Here's how the part is built. I have some questions about the finished solid (model axes, mm). A direction names the side the tool comes from. Coordinates: 2 decimals unless noted, no trailing zeros. Write each loop counter-clockwise with the first axis right and the second up, starting at its lowest first coordinate (ties: lowest second). Pieces come first, ordered by that corner, then holes.
(1) Imagine slicing it at B-B, the plane y = 72. List the corners of the cut face in (x, z) for me, plus the area to 3 significant figures.
(2) Imagine slicing it at A-A, the plane z = -4. List the corners of the cut face in (x, y) for me.
(3) Thinking about a two-plate mould opening in Y: for faces 1 (the cylindrical face through (-15.07, -64.7, 2.99)), 2 (the flat face through (-20, -18, -4)), 3 (the flat face through (15, -40, -6)), which applies, released by +Y, released by -Y, zero draft, split by the parting line, or undercut?
(4) For pin 1 Ø3 at (x, y) = (-17, -43) entering from -Z; pin 2 Ø20 at (x, y) = (-9.5, 35) entering from -Z; pin 3 Ø3 at (x, z) = (-5.5, -50.5) entering from -Y, each with a flat end and sliding along its axis, tell me the tip position at first contact or that it passes through.
(5) Imagine slicing it at C-C, the plane x = 0. List the corners of the cut face in (y, z) for me, plus the area to 3 significant figures.
(6) Imagine slicing it at D-D, the plane z = -20. List the corners of the cut face in (x, y) for me.
(7) Which directions (+Z, -Z, +X, -X, +Y, -Y) give clear straight access to the entire face, cutting with the end or side of a thin tool? Please do faces 4 (the flat face through (2, 55, 9)), 5 (the flat face through (20, -19, -4)), 6 (the flat face through (-10, -35.5, -6.4)), 7 (the flat face through (15, -41, 6)), 8 (the cylindrical face through (0, 20, 10)).
(8) Please list where these lines run through material, in increasing order: probe 1 along X at (y, z) = (0, -31); probe 2 along X at (y, z) = (-8, 4).
```python
from build123d import *

# Parameters (mm, degrees)
BOSS_EXTRUDE1_DEPTH      = 9
BOSS_EXTRUDE2_DEPTH      = 6
BOSS_EXTRUDE3_DEPTH      = 15
BOSS_EXTRUDE3_DEPTH_BACK = 70
SKETCH1_4_R              = 20
BOSS_EXTRUDE4_DEPTH      = 10
SKETCH3_W                = 10
SKETCH3_H                = 85.001


with BuildPart() as part:
    # Sketch1 → Boss-Extrude1 (new, symmetric)
    with BuildSketch(Plane.XY):
        with BuildLine():
            ThreePointArc((-29.862613088, 88), (2.137386912, 56), (34.137386912, 88))
            Line((34.137386912, 88), (42.137386912, 88))
            ThreePointArc((42.137386912, 88), (2.137386912, 48), (-37.862613088, 88))
            Line((-37.862613088, 88), (-29.862613088, 88))
        make_face()
    extrude(amount=BOSS_EXTRUDE1_DEPTH, both=True)

    # Sketch1<3> → Boss-Extrude2 (add, symmetric)
    with BuildSketch(Plane.XY):
        with BuildLine():
            ThreePointArc((20, 52.209958736), (-0.332230393, 48.076310411), (-20, 54.684296485))
            Line((-20, 54.684296485), (-20, 0))
            ThreePointArc((-20, 0), (0, 20), (20, 0))
            Line((20, 0), (20, 52.209958736))
        make_face()
    extrude(amount=BOSS_EXTRUDE2_DEPTH, both=True)

    # Sketch1<4> → Boss-Extrude3 (add, two sides: drawn at the far end of the back side and taken through both)
    with BuildSketch(Plane.XY.offset(-BOSS_EXTRUDE3_DEPTH_BACK)):
        Circle(SKETCH1_4_R)
    extrude(amount=BOSS_EXTRUDE3_DEPTH + BOSS_EXTRUDE3_DEPTH_BACK)

    # Sketch2 → Boss-Extrude4 (add)
    with BuildSketch(Plane(origin=(20, 0, 0), x_dir=(0, 0, -1), z_dir=(1, 0, 0))):
        with BuildLine():
            Line((-15, 0), (-15, -50))
            ThreePointArc((-15, -50), (-2.703242507, -64.754405442), (14.025663993, -55.317964795))
            Line((14.025663993, -55.317964795), (35, 0))
            Line((35, 0), (-15, 0))
        make_face()
        with BuildLine():
            Line((-6, -50), (-6, -31))
            ThreePointArc((-6, -31), (0, -25), (6, -31))
            Line((6, -31), (6, -50))
            ThreePointArc((6, -50), (0, -56), (-6, -50))
        make_face(mode=Mode.SUBTRACT)
    boss_extrude4 = extrude(amount=-BOSS_EXTRUDE4_DEPTH)

    # Mirror1: Boss-Extrude4 across plane
    add(boss_extrude4.mirror(Plane(origin=(0, 0, 0), x_dir=(0, 0, 1), z_dir=(1, 0, 0))))

    # Sketch3 → Ø20.0 (20) Diameter Hole1 (revolve, cut)
    with BuildSketch(Plane(origin=(0, 0, 15), x_dir=(0, -1, 0), z_dir=(1, 0, 0))):
        with Locations((5, 42.5005)):
            Rectangle(SKETCH3_W, SKETCH3_H)
    revolve(axis=Axis((0, 0, 21.35), (0, 0, -1)), mode=Mode.SUBTRACT)


solid = part.part
```
Recorded:
1. outline: (-34.52, -9) - (-25.58, -9) - (-25.58, 9) - (-34.52, 9) - close; (29.85, -9) - (38.8, -9) - (38.8, 9) - (29.85, 9) - close
1. area: 322 mm2
2. outline: (-37.86, 88) arc R40 ccw to (-20, 54.68) - (-20, -26.53) - (-10, -26.53) - (-10, -17.32) arc R20 ccw to (10, -17.32) - (10, -26.53) - (20, -26.53) - (20, 52.21) arc R40 ccw to (42.14, 88) - (34.14, 88) arc R32 cw to (-29.86, 88) - close; (-20, -64.46) - (-10, -64.46) - (-10, -54.47) - (-20, -54.47) - close; (10, -64.46) - (20, -64.46) - (20, -54.47) - (10, -54.47) - close; hole circle Ø20 at (0, 0)
3. face 1: released by -Y
3. face 2: zero draft
3. face 3: undercut
4. pin 1: stops at z = -19.26
4. pin 2: stops at z = -6
4. pin 3: stops at y = -19.6
5. outline: (-20, -70) - (-10, -70) - (-10, 15) - (-20, 15) - close; (10, -70) - (20, -70) - (20, -6) - (48.06, -6) - (48.06, -9) - (56.07, -9) - (56.07, 9) - (48.06, 9) - (48.06, 6) - (20, 6) - (20, 15) - (10, 15) - close
5. area: 2,180 mm2
6. outline: (-20, -39.56) - (-10, -39.56) - (-10, -17.32) arc R20 ccw to (10, -17.32) - (10, -39.56) - (20, -39.56) - (20, 0) arc R20 ccw to (-20, 0) - close; hole circle Ø20 at (0, 0)
7. face 4: +Z, +X, -X, +Y
7. face 5: +Z, -Z, +X, -Y
7. face 6: +Z, -Z, -Y
7. face 7: +X, -X
7. face 8: +Z
8. probe 1: x = -20 to -10, 10 to 20
8. probe 2: x = -20 to -6, 6 to 20
